from build123d import *

# Parameters (mm, degrees)
SKETCH_W        = 98
SKETCH_H        = 52
PAD_DEPTH       = 9.3
SKETCH001_W     = 20
SKETCH001_H     = 5
POCKET_DEPTH    = 9.301
SKETCH002_W     = 15
SKETCH002_H     = 14.666667
SKETCH002_H_2   = 14.666666
SKETCH002_W_2   = 26
SKETCH002_H_3   = 48
SKETCH002_H_4   = 11.333333
SKETCH002_H_5   = 11.333334
POCKET001_DEPTH = 7


with BuildPart() as part:
    # Sketch → Pad (new body)
    with BuildSketch(Plane.XY):
        with Locations((49, 26)):
            Rectangle(SKETCH_W, SKETCH_H)
    extrude(amount=PAD_DEPTH)

    # Sketch001 (on Face6 of Pad) → Pocket (cut, through all)
    with BuildSketch(Plane.XY.offset(9.3)):
        with Locations((88, 49.5)):
            Rectangle(SKETCH001_W, SKETCH001_H)
        with Locations((88, 2.5)):
            Rectangle(SKETCH001_W, SKETCH001_H)
    extrude(amount=-POCKET_DEPTH, mode=Mode.SUBTRACT)

    # Sketch002 (on Face6 of Pad) → Pocket001 (cut)
    with BuildSketch(Plane.XY.offset(9.3)):
        with Locations((9.5, 42.666666)):
            Rectangle(SKETCH002_W, SKETCH002_H)
        with Locations((9.5, 26)):
            Rectangle(SKETCH002_W, SKETCH002_H_2)
        with Locations((9.5, 9.333334)):
            Rectangle(SKETCH002_W, SKETCH002_H)
        with Locations((26.5, 42.666666)):
            Rectangle(SKETCH002_W, SKETCH002_H)
        with Locations((26.5, 26)):
            Rectangle(SKETCH002_W, SKETCH002_H_2)
        with Locations((26.5, 9.333334)):
            Rectangle(SKETCH002_W, SKETCH002_H)
        with Locations((49, 26)):
            Rectangle(SKETCH002_W_2, SKETCH002_H_3)
        with Locations((71.5, 39.371451)):
            Rectangle(SKETCH002_W, SKETCH002_H_4)
        with Locations((71.5, 26.038118)):
            Rectangle(SKETCH002_W, SKETCH002_H_5)
        with Locations((71.5, 12.704785)):
            Rectangle(SKETCH002_W, SKETCH002_H_4)
        with Locations((88.5, 39.371451)):
            Rectangle(SKETCH002_W, SKETCH002_H_4)
        with Locations((88.5, 26.038118)):
            Rectangle(SKETCH002_W, SKETCH002_H_5)
        with Locations((88.5, 12.704785)):
            Rectangle(SKETCH002_W, SKETCH002_H_4)
    extrude(amount=-POCKET001_DEPTH, mode=Mode.SUBTRACT)


solid = part.part
Design review of the part built by this model. Coordinates are the model's own, in mm. Coordinates: 2 decimals unless noted, no trailing zeros. Write each loop counter-clockwise with the first axis right and the second up, starting at its lowest first coordinate (ties: lowest second). Pieces come first, ordered by that corner, then holes. Notation, with made-up numbers: (35.5, 33) -> (84.5, 33) arc R35 cw to (84.5, 69) -> close; hole circle Ø9 at (27, -23.75). An arc over 180 degrees is marked (long way). Write each question's results on one line, items separated by ' | '. Start each with the question number.
(1) The part is to be moulded in two halves that separate along Y. For faces 1 (the face through (88, 47, 5)), 2 (the face through (26, 18.667, 6)), say which applies: pulls with the +Y half, pulls with the -Y half, needs draft (parallel to the pull), parting line crosses it, or undercut.
(2) Take a section at B-B on y = 48.5. Write out the cut boundary in (x, z).
(3) Take a section at D-D on x = 67.5. Write out the cut boundary in (y, z).
(4) Take a section at A-A on x = 40. Write out the cut boundary in (y, z), and give its area (3 significant figures).
(5) For line 1 along X through (y, z) = (3, 7); line 2 along Y through (x, z) = (23, 8.25); line 3 along X through (y, z) = (17, 7.25), list the stretches that pass through material, from the lowest coordinate up. Write a range as from..to.
(6) Take a section at C-C on z = 5. Give the number of separate pieces and of enclosed holes in the cut face, and give its area (3 significant figures).
(7) Clearance check with flat-ended pins moving along their axes: P1, Ø4, axis at x = 60.5, y = 41, coming from the -Z side; P2, Ø3.5, axis at x = 72.5, y = 13, coming from the +Z side; P3, Ø4.5, axis at x = 89.5, z = 4.5, coming from the -Y side. State where each tip first meets the part, or that it passes through.
Results found:
1) face 1: pulls with the +Y half | face 2: undercut
2) outline: (0, 0) -> (78, 0) -> (78, 9.3) -> (62, 9.3) -> (62, 2.3) -> (36, 2.3) -> (36, 9.3) -> (34, 9.3) -> (34, 2.3) -> (19, 2.3) -> (19, 9.3) -> (17, 9.3) -> (17, 2.3) -> (2, 2.3) -> (2, 9.3) -> (0, 9.3) -> close
3) outline: (0, 0) -> (52, 0) -> (52, 9.3) -> (45.04, 9.3) -> (45.04, 2.3) -> (33.7, 2.3) -> (33.7, 9.3) -> (31.7, 9.3) -> (31.7, 2.3) -> (20.37, 2.3) -> (20.37, 9.3) -> (18.37, 9.3) -> (18.37, 2.3) -> (7.04, 2.3) -> (7.04, 9.3) -> (0, 9.3) -> close
4) outline: (0, 0) -> (52, 0) -> (52, 9.3) -> (50, 9.3) -> (50, 2.3) -> (2, 2.3) -> (2, 9.3) -> (0, 9.3) -> close | area: 148 mm2
5) line 1: x = 0..2, 17..19, 34..36, 62..78 | line 2: y = 0..2, 16.67..18.67, 33.33..35.33, 50..52 | line 3: x = 0..36, 62..64, 79..81, 96..98
6) separate pieces: 1 | enclosed holes: 13 | area: 1,310 mm2
7) P1: stops at z = 0 | P2: stops at z = 2.3 | P3: stops at y = 5
